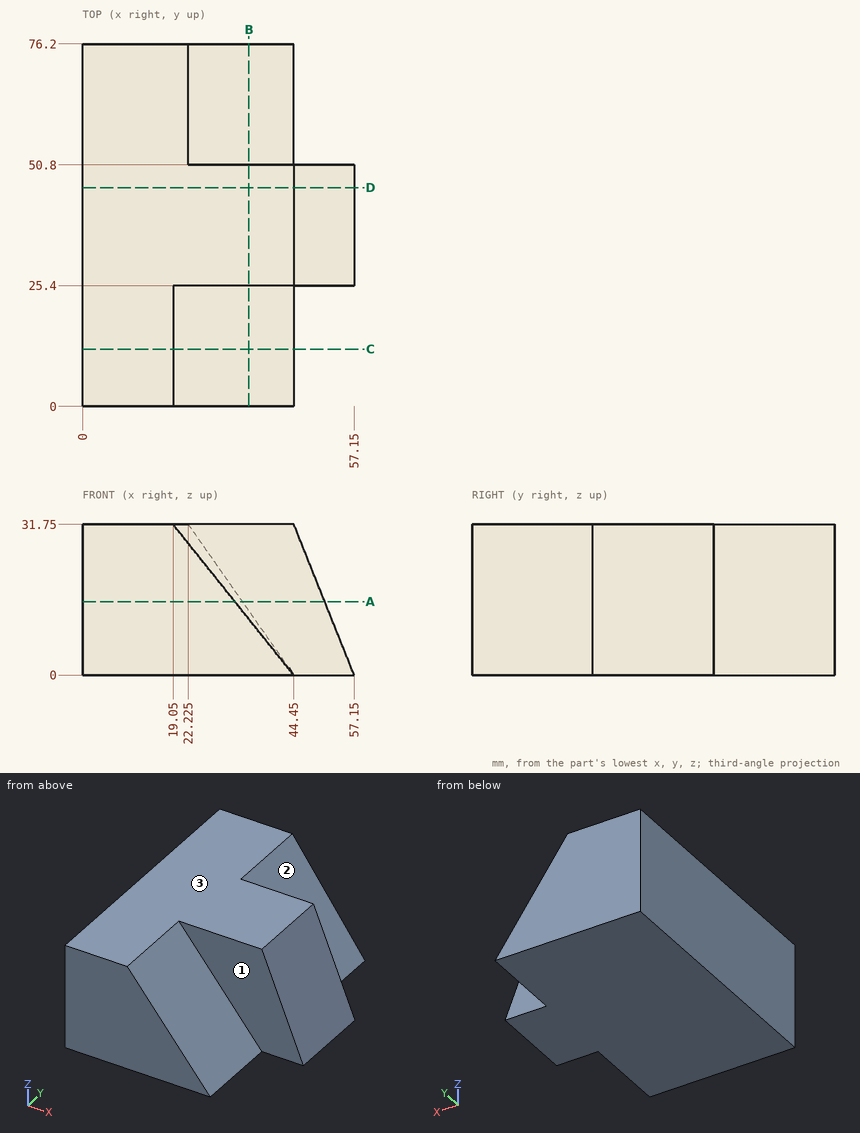
Can you work these out from the drawing? Everything is in mm from the part's minimum corner. A direction names the side the tool comes from. Round coordinates to 2 decimals unless told otherwise and drop trailing zeros. Loops run counter-clockwise (first coordinate to the right, second up) from the corner with the lowest first, then second, coordinate; pieces in that order, holes last.
1. If we section it at B-B on x = 35: Write out the boundary of the cut face in (y, z).
Answer list:
outline: (0, 0) - (76.2, 0) - (76.2, 13.5) - (50.8, 13.5) - (50.8, 31.75) - (25.4, 31.75) - (25.4, 11.81) - (0, 11.81) - close
2. For P1, Ø1.5, axis at y = 13.5, z = 16.5, coming from the +X side; P2, Ø6, axis at y = 53, z = 25.5, coming from the +X side; P3, Ø1.5, axis at x = 31, y = 53, coming from the +Z side, each with a flat end and sliding along its axis, tell me the tip position at first contact or that it passes through.
Answer list:
P1: stops at x = 31.85
P2: stops at x = 47.77
P3: stops at z = 20.29
3. If we section it at A-A on z = 15.5: Write out the boundary of the cut face in (x, y).
Answer list:
outline: (0, 0) - (32.05, 0) - (32.05, 25.4) - (50.95, 25.4) - (50.95, 50.8) - (33.6, 50.8) - (33.6, 76.2) - (0, 76.2) - close
4. If we section it at C-C on y = 12: Write out the boundary of the cut face in (x, z), plus the area to 3 significant figures.
Answer list:
outline: (0, 0) - (44.45, 0) - (19.05, 31.75) - (0, 31.75) - close
area: 1,010 mm2
5. Which directions (+Z, -Z, +X, -X, +Y, -Y) give clear straight access to the entire face, cutting with the end or side of a thin tool? Please do the marked faces 1, 2 and 3.
Answer list:
face 1: +Z, +X, -Y
face 2: +Z, +X, +Y
face 3: +Z, +X, -X, +Y, -Y
6. If we section it at D-D on y = 46: Write out the boundary of the cut face in (x, z).
Answer list:
outline: (0, 0) - (57.15, 0) - (44.45, 31.75) - (0, 31.75) - close
7. If I drill on line 1 along Y through (x, z) = (43, 11.5); line 2 along X through (y, z) = (7.5, 26); line 3 along X through (y, z) = (37, 11), over which ranges is the centre line in solid material (lowest first)?
Answer list:
line 1: y = 25.4 to 50.8
line 2: x = 0 to 23.65
line 3: x = 0 to 52.75
